Check sheet for the modelled part. Datum: model origin and axes. Units: mm. Coordinates: 2 decimals unless noted, no trailing zeros. Loops run counter-clockwise (first coordinate to the right, second up) from the corner with the lowest first, then second, coordinate; pieces in that order, holes last. Notation, with made-up numbers: (84.5, -11.5) - (127.5, -11.5) arc R17 ccw to (127.5, -6.5) - close; hole circle Ø3 at (51.25, 67). An arc over 180 degrees is marked (long way). Use a Markdown table: item, result. Add a question column.
1) Sectioned sample at B-B, the plane x = 0. Enter the section's corners in (y, z), then the cut area to 3 significant figures.
2) Sectioned sample at A-A, the plane x = -57. Enter the section's corners in (y, z).
3) Sectioned sample at D-D, the plane z = 1.5. State how many separate pieces and enclosed holes the cut face has, then the cut area to 3 significant figures.
4) Sectioned sample at C-C, the plane x = -33.5. Enter the section's corners in (y, z), then the cut area to 3 significant figures.
5) Go/stop test with a flat-tipped pin: P1, Ø4, axis at x = -36.5, y = 6, coming from the +Z side. Record where the tip stops, or that it passes through.
6) Thickness scan on line 1 (Y direction, x = -57, z = 1.15); line 2 (Y direction, x = -25, z = 0.6); line 3 (Y direction, x = -28, z = 0.7). Record the ranges inside material, lowest first.
7) Draft check along X on faces 1 (the flat face through (-39.032, -2.712, 1.014)), 2 (the flat face through (1, 15, 2)). Enter one of: pulls with the +X half, pulls with the -X half, needs draft (parallel to the pull), parting line crosses it, or undercut.
from build123d import *

# Parameters (mm, degrees)
SKETCH_1_W          = 130
SKETCH_1_H          = 43
EXTRUDE_1_DEPTH     = 2
CUT_EXTRUDE_1_DEPTH = 69.492700341
SKETCH_3_R          = 1.7
CUT_EXTRUDE_2_DEPTH = 69.492700341
SKETCH_4_R          = 10
SKETCH_4_W          = 34
SKETCH_4_H          = 35
CUT_EXTRUDE_3_DEPTH = 69.492700341
EXTRUDE_2_DEPTH     = 2


with BuildPart() as part:
    # 草图1 → 凸台-拉伸1 (new body)
    with BuildSketch(Plane.XY):
        Rectangle(SKETCH_1_W, SKETCH_1_H)
    extrude(amount=EXTRUDE_1_DEPTH)

    # 草图2 → 切除-拉伸1 (cut, through all)
    with BuildSketch(Plane.XY.offset(2)):
        with BuildLine():
            Line((-12.585786438, 15.414213562), (-10.110912703, 12.939339828))
            ThreePointArc((-10.110912703, 12.939339828), (-10.110912703, 10.110912703), (-12.939339828, 10.110912703))
            Line((-12.939339828, 10.110912703), (-15.414213562, 12.585786438))
            ThreePointArc((-15.414213562, 12.585786438), (-15.414213562, 15.414213562), (-12.585786438, 15.414213562))
        make_face()
        with BuildLine():
            Line((15.414213562, 12.585786438), (12.939339828, 10.110912703))
            ThreePointArc((12.939339828, 10.110912703), (10.110912703, 10.110912703), (10.110912703, 12.939339828))
            Line((10.110912703, 12.939339828), (12.585786438, 15.414213562))
            ThreePointArc((12.585786438, 15.414213562), (15.414213562, 15.414213562), (15.414213562, 12.585786438))
        make_face()
        with BuildLine():
            Line((12.585786438, -15.414213562), (10.110912703, -12.939339828))
            ThreePointArc((10.110912703, -12.939339828), (10.110912703, -10.110912703), (12.939339828, -10.110912703))
            Line((12.939339828, -10.110912703), (15.414213562, -12.585786438))
            ThreePointArc((15.414213562, -12.585786438), (15.414213562, -15.414213562), (12.585786438, -15.414213562))
        make_face()
        with BuildLine():
            Line((-15.414213562, -12.585786438), (-12.939339828, -10.110912703))
            ThreePointArc((-12.939339828, -10.110912703), (-10.110912703, -10.110912703), (-10.110912703, -12.939339828))
            Line((-10.110912703, -12.939339828), (-12.585786438, -15.414213562))
            ThreePointArc((-12.585786438, -15.414213562), (-15.414213562, -15.414213562), (-15.414213562, -12.585786438))
        make_face()
    extrude(amount=-CUT_EXTRUDE_1_DEPTH, mode=Mode.SUBTRACT)

    # 草图3 → 切除-拉伸2 (cut, through all)
    with BuildSketch(Plane.XY.offset(2)):
        with Locations((57, 5)):
            Circle(SKETCH_3_R)
        with Locations((57, -5)):
            Circle(SKETCH_3_R)
        with Locations(Location((-57, -5, 0), (0, 0, 180))):
            Circle(SKETCH_3_R)
        with Locations(Location((-57, 5, 0), (0, 0, 180))):
            Circle(SKETCH_3_R)
    extrude(amount=-CUT_EXTRUDE_2_DEPTH, mode=Mode.SUBTRACT)

    # 草图4 → 切除-拉伸3 (cut, through all)
    with BuildSketch(Plane.XY.offset(2)):
        Circle(SKETCH_4_R)
        with Locations((-36, 0)):
            Rectangle(SKETCH_4_W, SKETCH_4_H)
        with Locations((36, 0)):
            Rectangle(SKETCH_4_W, SKETCH_4_H)
    extrude(amount=-CUT_EXTRUDE_3_DEPTH, mode=Mode.SUBTRACT)

    # 草图6 → 凸台-拉伸2 (add, through all)
    with BuildSketch(Plane.XY.offset(2)):
        Polygon((-19, -17.5), (-53, 17.5), (-53, 11.666666667), (-24.666666667, -17.5), align=None)
        Polygon((-41.666666667, 17.5), (-47.333333333, 17.5), (-19, -11.666666667), (-19, -5.833333333), align=None)
        Polygon((-30.333333333, -17.5), (-53, 5.833333333), (-53, 0), (-36, -17.5), align=None)
        Polygon((-30.333333333, 17.5), (-36, 17.5), (-19, 0), (-19, 5.833333333), align=None)
        Polygon((-41.666666667, -17.5), (-53, -5.833333333), (-53, -11.666666667), (-47.333333333, -17.5), align=None)
        Polygon((-19, 17.5), (-24.666666667, 17.5), (-19, 11.666666667), align=None)
    extrude_2 = extrude(amount=-EXTRUDE_2_DEPTH)

    # 镜向1: 凸台-拉伸2 across plane
    add(extrude_2.mirror(Plane(origin=(0, 0, 0), x_dir=(0, 0, 1), z_dir=(1, 0, 0))))


solid = part.part
Solved:
| question | item | result |
|---|---|---|
| 1 | outline | (-21.5, 0) - (-10, 0) - (-10, 2) - (-21.5, 2) - close; (10, 0) - (21.5, 0) - (21.5, 2) - (10, 2) - close |
| 1 | area | 46.0 mm2 |
| 2 | outline | (-21.5, 0) - (-6.7, 0) - (-6.7, 2) - (-21.5, 2) - close; (-3.3, 0) - (3.3, 0) - (3.3, 2) - (-3.3, 2) - close; (6.7, 0) - (21.5, 0) - (21.5, 2) - (6.7, 2) - close |
| 3 | separate pieces | 1 |
| 3 | enclosed holes | 21 |
| 3 | area | 3,940 mm2 |
| 4 | outline | (-21.5, 0) - (-14.24, 0) - (-14.24, 2) - (-21.5, 2) - close; (-8.41, 0) - (-2.57, 0) - (-2.57, 2) - (-8.41, 2) - close; (3.26, 0) - (9.09, 0) - (9.09, 2) - (3.26, 2) - close; (14.93, 0) - (21.5, 0) - (21.5, 2) - (14.93, 2) - close |
| 4 | area | 51.0 mm2 |
| 5 | P1 | stops at z = 2 |
| 6 | line 1 | y = -21.5 to -6.7, -3.3 to 3.3, 6.7 to 21.5 |
| 6 | line 2 | y = -21.5 to -17.5, -17.16 to -11.32, -5.49 to 0.34, 6.18 to 12.01, 17.5 to 21.5 |
| 6 | line 3 | y = -21.5 to -17.5, -14.07 to -8.24, -2.4 to 3.43, 9.26 to 15.1, 17.5 to 21.5 |
| 7 | face 1 | undercut |
| 7 | face 2 | needs draft |
